For this review, take the finished solid that the model builds, in its own axes (mm). Round coordinates to 2 decimals unless told otherwise and drop trailing zeros. Write each loop counter-clockwise with the first axis right and the second up, starting at its lowest first coordinate (ties: lowest second). Pieces come first, ordered by that corner, then holes. Notation, with made-up numbers: M -25.75,-14 L 19.25,-14 A33 cw 19.25,21 Z; hole C 86.25,-19 d2. An arc over 180 degrees is marked long. Use one line per item in the form item = value. Start each with the question number.
Item 1: For P1, Ø5, axis at x = 84.5, y = 9, coming from the -Z side; P2, Ø8, axis at x = -235, y = 0.5, coming from the -Z side; P3, Ø12.5, axis at y = -5.5, z = -128, coming from the -X side, all flat-tipped, find the tip position at first contact; note any pin that passes through.
Item 2: Add section A-A (y = 0.5). State the section outline as (x, z) points.
Item 3: Add section B-B (z = -228.5). State the section outline as (x, y) points.
Item 4: For line 1 (Z direction, x = -1326, y = 5); line 2 (Z direction, x = -491.5, y = 10); line 3 (Z direction, x = 615, y = 3.25), list the stretches that pass through material, from the lowest coordinate up. Write a range as [from, to].
Item 5: Add section C-C (x = -130). State the section outline as (y, z) points.
Item 6: Add section D-D (x = 791.5). State the section outline as (y, z) points, and give its area (3 significant figures).
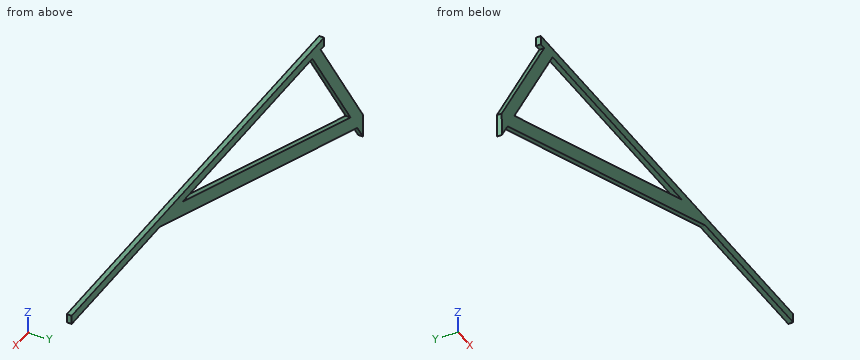
from build123d import *

# Parameters (mm, degrees)
F1_DEPTH = 12.7


with BuildPart() as f1:
    # F0 (on Front) → F1 (new body, symmetric)
    with BuildSketch(Plane.XZ):
        Polygon((-598.979303, -141.286989), (-598.979303, -94.24994), (-1076.970816, -94.24994), (-1076.970816, -142.254412), (-1044.996943, -142.254412), (-966.876544, -142.254412), (-966.272031, -141.286989), align=None)
        Polygon((1306.020697, -94.24994), (-598.979303, -94.24994), (-598.979303, -141.286989), (256.845117, -141.286989), (475.207098, -141.286989), (1306.020697, -141.286989), align=None)
        Polygon((475.207098, -141.286989), (256.845117, -141.286989), (-1326.34247, -717.520147), (-1390.625515, -820.394523), align=None)
        Polygon((-1390.625515, -820.394523), (-1326.34247, -717.520147), (-966.876544, -142.254412), (-1044.996943, -142.254412), (-1446.578518, -784.919273), (-1443.203137, -904.536307), align=None)
    extrude(amount=F1_DEPTH, both=True)


solid = f1.part
Calculated:
q1.P1 = -284.4
q1.P2 = -401.24
q1.P3 = -1076.97
q2.outline = M -1446.58,-784.92 L -1443.2,-904.54 L -1390.63,-820.39 L 475.21,-141.29 L 1306.02,-141.29 L 1306.02,-94.25 L -1076.97,-94.25 L -1076.97,-142.25 L -1045,-142.25 Z; hole M -1326.34,-717.52 L 256.85,-141.29 L -966.27,-141.29 Z
q3.outline = M -1098.89,-12.7 L -1020.77,-12.7 L -1020.77,12.7 L -1098.89,12.7 Z; M 17.23,-12.7 L 235.59,-12.7 L 235.59,12.7 L 17.23,12.7 Z
q4.line_1 = [-796.87, -717.4], [-716.97, -591.95]
q4.line_2 = [-493.14, -413.66], [-141.29, -94.25]
q4.line_3 = [-141.29, -94.25]
q5.outline = M -12.7,-361.56 L 12.7,-361.56 L 12.7,-282.09 L -12.7,-282.09 Z; M -12.7,-141.29 L 12.7,-141.29 L 12.7,-94.25 L -12.7,-94.25 Z
q6.outline = M -12.7,-141.29 L 12.7,-141.29 L 12.7,-94.25 L -12.7,-94.25 Z
q6.area = 1,190 mm^2
